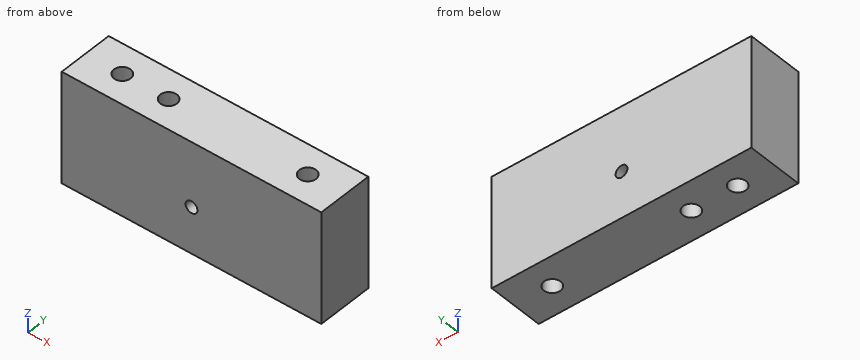
from build123d import *

# Parameters (mm, degrees)
SKETCH1_W           = 140
SKETCH1_H           = 60
BOSS_EXTRUDE1_DEPTH = 30
SKETCH2_R           = 4.5
CUT_EXTRUDE1_DEPTH  = 60
SKETCH3_R           = 3.2
CUT_EXTRUDE2_DEPTH  = 30


with BuildPart() as part:
    # Sketch1 → Boss-Extrude1 (new body)
    with BuildSketch(Plane(origin=(0, 0, 0), x_dir=(1, 0, 0), z_dir=(0, 1, 0))):
        Rectangle(SKETCH1_W, SKETCH1_H)
    extrude(amount=BOSS_EXTRUDE1_DEPTH)

    # Sketch2 → Cut-Extrude1 (cut)
    with BuildSketch(Plane.XY.offset(30)):
        with Locations((50, 15)):
            Circle(SKETCH2_R)
        with Locations((-50, 15)):
            Circle(SKETCH2_R)
        with Locations((-25, 15)):
            Circle(SKETCH2_R)
    extrude(amount=-CUT_EXTRUDE1_DEPTH, mode=Mode.SUBTRACT)

    # Sketch3 → Cut-Extrude2 (cut)
    with BuildSketch(Plane(origin=(0, 30, 0), x_dir=(1, 0, 0), z_dir=(0, 1, 0))):
        with Locations(Location((0, 5, 0), (0, 0, 270))):
            Circle(SKETCH3_R)
    extrude(amount=-CUT_EXTRUDE2_DEPTH, mode=Mode.SUBTRACT)


solid = part.part
Input: part model. Units: mm. Frame: model coordinates. Give positions to 0.01 mm unless a question says otherwise; leave off trailing zeros. Order: outer loops, then holes, each group sorted by start corner. A loop starts at its lowest first (then second) coordinate and runs counter-clockwise, first axis right, second up. Notation, with made-up numbers: (73.5, 67) -> (80.5, 67) arc R18 ccw to (80.5, 95) -> close; hole circle Ø5 at (71, 21.25). An arc over 180 degrees is marked (long way). Use one line per item in the form item = value.
1) First-contact query: pin 1 Ø5.5 at (x, y) = (-50, 15) entering from +Z. Flat tip, straight axial feed; report the tip coordinate or a pass-through.
Response values:
pin_1 = through
2) Section A-A, the plane y = 15. Return loops of the section in (x, z).
Response values:
outline = (-70, -30) -> (-54.5, -30) -> (-54.5, 30) -> (-70, 30) -> close; (-45.5, -30) -> (-29.5, -30) -> (-29.5, 30) -> (-45.5, 30) -> close; (-20.5, -30) -> (45.5, -30) -> (45.5, 30) -> (-20.5, 30) -> close; (54.5, -30) -> (70, -30) -> (70, 30) -> (54.5, 30) -> close; hole circle Ø6.4 at (0, -5)
3) Line query: probe 1 along Y at (x, z) = (-50, -16); probe 2 along X at (y, z) = (17.25, -5); probe 3 along X at (y, z) = (17.5, -5). Output: solid intervals per line, ascending.
Response values:
probe_1 = 0 to 10.5, 19.5 to 30
probe_2 = -70 to -53.9, -46.1 to -28.9, -21.1 to -3.2, 3.2 to 46.1, 53.9 to 70
probe_3 = -70 to -53.74, -46.26 to -28.74, -21.26 to -3.2, 3.2 to 46.26, 53.74 to 70
4) Section B-B, the plane z = -5. Return loops of the section in (x, y), and give its area (3 significant figures).
Response values:
outline = (-70, 0) -> (-3.2, 0) -> (-3.2, 30) -> (-70, 30) -> close; (3.2, 0) -> (70, 0) -> (70, 30) -> (3.2, 30) -> close; hole circle Ø9 at (-50, 15); hole circle Ø9 at (-25, 15); hole circle Ø9 at (50, 15)
area = 3,820 mm^2
5) Section D-D, the plane z = 3. Return loops of the section in (x, y), and give its area (3 significant figures).
Response values:
outline = (-70, 0) -> (70, 0) -> (70, 30) -> (-70, 30) -> close; hole circle Ø9 at (-50, 15); hole circle Ø9 at (-25, 15); hole circle Ø9 at (50, 15)
area = 4,010 mm^2
6) Section C-C, the plane x = 0. Return loops of the section in (y, z).
Response values:
outline = (0, -30) -> (30, -30) -> (30, -8.2) -> (0, -8.2) -> close; (0, -1.8) -> (30, -1.8) -> (30, 30) -> (0, 30) -> close
